The listing builds one solid part. Answer for the finished solid, in the listing's coordinates (mm). Round coordinates to 2 decimals unless told otherwise and drop trailing zeros. Write each loop counter-clockwise with the first axis right and the second up, starting at its lowest first coordinate (ties: lowest second). Pieces come first, ordered by that corner, then holes. Notation, with made-up numbers: (7, 47.5) - (38, 47.5) arc R37 ccw to (38, 85.5) - close; hole circle Ø11 at (-36.5, 81.25). An arc over 180 degrees is marked (long way). Return JSON: item names as keys, results as strings. Group by question number.
(1) Find the intervals of material crossed by line 1 along Z through (x, y) = (5, 3); line 2 along X through (y, z) = (2.5, -13); line 3 along Z through (x, y) = (-9, 6), in increasing order. Write a range as [from, to].
(2) Section B-B, the plane x = -13 is taken. Write down the section's boundary in (y, z), then the cut area to 3 significant figures.
(3) This flat-tipped pin is pushed along its axis until it touches: pin 1 (1.5 mm diameter, centred on x = -9.5, y = 5, fed in from +Z). Where does it stop, or does it pass through?
(4) Section C-C, the plane z = 5.5 is taken. Write down the section's boundary in (x, y).
(5) Section A-A, the plane y = 3 is taken. Write down the section's boundary in (x, z).
```python
from build123d import *

# Parameters (mm, degrees)
SKETCH1_R           = 19.05
BOSS_EXTRUDE1_DEPTH = 6.35
BOSS_EXTRUDE2_DEPTH = 6.35
FILLET13_R          = 1.27
FILLET15_R          = 1.27


with BuildPart() as part:
    # Sketch1 → Boss-Extrude1 (new body)
    with BuildSketch(Plane(origin=(0, 0, 0), x_dir=(1, 0, 0), z_dir=(0, 1, 0))):
        with Locations(Location((0, 0, 0), (0, 0, 270))):
            Circle(SKETCH1_R)
    extrude(amount=BOSS_EXTRUDE1_DEPTH)

    # Sketch2 → Boss-Extrude2 (add)
    with BuildSketch(Plane(origin=(0, 0, 0), x_dir=(1, 0, 0), z_dir=(0, 1, 0))):
        Polygon((-2.992120362, 18.813551386), (-2.286000743, 23.480131449), (2.285999257, 23.480131449), (2.992119638, 18.813551501), align=None)
    extrude(amount=BOSS_EXTRUDE2_DEPTH)

    # Fillet13
    fillet13_edges = [part.edges().sort_by_distance(p)[0] for p in [
        (2.285999257, 3.175, -23.480131449),
        (-2.286000743, 3.175, -23.480131449),
        (-7.43e-07, 0, -23.480131449),
        (-7.43e-07, 6.35, -23.480131449),
    ]]
    fillet(fillet13_edges, radius=FILLET13_R)

    # Fillet15
    fillet15_edges = [part.edges().sort_by_distance(p)[0] for p in [
        (-2.992120362, 3.175, -18.813551386),
        (2.992119638, 3.175, -18.813551501),
    ]]
    fillet(fillet15_edges, radius=FILLET15_R)


solid = part.part
```
Working result:
{
 "1": {"line 1": "z = [-18.38, 18.38]", "line 2": "x = [-13.92, 13.92]", "line 3": "z = [-16.79, 16.79]"},
 "2": {"outline": "(0, -13.92) - (6.35, -13.92) - (6.35, 13.92) - (0, 13.92) - close", "area": "177 mm^2"},
 "3": {"pin 1": "stops at z = 16.92"},
 "4": {"outline": "(-18.24, 0) - (18.24, 0) - (18.24, 6.35) - (-18.24, 6.35) - close"},
 "5": {"outline": "(-3.86, -18.66) arc R1.27 cw to (-2.86, -19.71) - (-2.45, -22.4) arc R1.27 ccw to (-1.19, -23.48) - (1.19, -23.48) arc R1.27 ccw to (2.45, -22.4) - (2.86, -19.71) arc R1.27 cw to (3.86, -18.66) arc R19.05 ccw (long way) to start"}
}
